Read the model definition and answer for the solid it produces. Units are mm, in the model's axes. Give positions to 0.01 mm unless a question says otherwise; leave off trailing zeros. Write each loop counter-clockwise with the first axis right and the second up, starting at its lowest first coordinate (ties: lowest second). Pieces come first, ordered by that corner, then holes. Notation, with made-up numbers: (-9.75, 11.5) -> (30.25, 11.5) arc R17 ccw to (30.25, 44.5) -> close; hole circle Ø4 at (19.25, 76). An arc over 180 degrees is marked (long way). Write item = value, one per line.
from build123d import *

# Parameters (mm, degrees)
F0_R     = 7.25
F1_DEPTH = 12.7


with BuildPart() as f1:
    # F0 (on Right) → F1 (new body)
    with BuildSketch(Plane.YZ):
        with BuildLine():
            Line((7.25, 21.75), (-7.25, 21.75))
            ThreePointArc((-7.25, 21.75), (-17.503048, 17.503048), (-21.75, 7.25))
            Line((-21.75, 7.25), (-21.75, -172.35))
            ThreePointArc((-21.75, -172.35), (-17.503048, -182.603048), (-7.25, -186.85))
            Line((-7.25, -186.85), (7.25, -186.85))
            ThreePointArc((7.25, -186.85), (17.503048, -182.603048), (21.75, -172.35))
            Line((21.75, -172.35), (21.75, 7.25))
            ThreePointArc((21.75, 7.25), (17.503048, 17.503048), (7.25, 21.75))
        make_face()
        with Locations((0, -165.1)):
            Circle(F0_R, mode=Mode.SUBTRACT)
        Circle(F0_R, mode=Mode.SUBTRACT)
    extrude(amount=F1_DEPTH)


solid = f1.part
(1) The part is cut by section B-B on y = -5.5. Determine the outline of the cut face in (x, z), plus the area to 3 significant figures.
Checks:
outline = (0, -186.85) -> (12.7, -186.85) -> (12.7, -169.82) -> (0, -169.82) -> close; (0, -160.38) -> (12.7, -160.38) -> (12.7, -4.72) -> (0, -4.72) -> close; (0, 4.72) -> (12.7, 4.72) -> (12.7, 21.75) -> (0, 21.75) -> close
area = 2,410 mm²
(2) The part is cut by section A-A on z = -165.1. Determine the outline of the cut face in (x, y), plus the area to 3 significant figures.
Checks:
outline = (0, -21.75) -> (12.7, -21.75) -> (12.7, -7.25) -> (0, -7.25) -> close; (0, 7.25) -> (12.7, 7.25) -> (12.7, 21.75) -> (0, 21.75) -> close
area = 368 mm²
(3) The part is cut by section D-D on y = 17.5. Determine the outline of the cut face in (x, z).
Checks:
outline = (0, -182.61) -> (12.7, -182.61) -> (12.7, 17.51) -> (0, 17.51) -> close
(4) Consider L1, parallel to Z at x = 5.25, y = 0; L2, parallel to Z at x = 7.5, y = 6; L3, parallel to Y at x = 1.75, z = -171.5. Determine where each line is inside the solid, lowest interval first.
Checks:
L1 = -186.85 to -172.35, -157.85 to -7.25, 7.25 to 21.75
L2 = -186.85 to -169.17, -161.03 to -4.07, 4.07 to 21.75
L3 = -21.75 to -3.41, 3.41 to 21.75
(5) The part is cut by section C-C on x = 3.5. Determine the outline of the cut face in (y, z).
Checks:
outline = (-21.75, -172.35) arc R14.5 ccw to (-7.25, -186.85) -> (7.25, -186.85) arc R14.5 ccw to (21.75, -172.35) -> (21.75, 7.25) arc R14.5 ccw to (7.25, 21.75) -> (-7.25, 21.75) arc R14.5 ccw to (-21.75, 7.25) -> close; hole circle Ø14.5 at (0, -165.1); hole circle Ø14.5 at (0, 0)
(6) For a pull along Z with two mould halves and no side action, classify faces 1 (the cylindrical face through (6.261, 17.615, 17.39)), 2 (the flat face through (6, 21.75, -84)), 3 (the cylindrical face through (6.26, 3.35, -6.43)) as released by +Z, released by -Z, zero draft, split by the parting line, or undercut.
Checks:
face_1 = released by +Z
face_2 = zero draft
face_3 = undercut
